```python
from build123d import *

# Parameters (mm, degrees)
F0_W          = 27
F0_H          = 27
F1_DEPTH      = 0.8
F2_D          = 2.65
F3_R          = 2
F4_W          = 5
F4_H          = 8
F4_W_2        = 8
F4_H_2        = 6
F4_R          = 0.9
F5_DEPTH      = 3
F7_DEPTH      = 2.8
F7_DEPTH_BACK = 2


with BuildPart() as f1:
    # F0 (on Top) → F1 (new body)
    with BuildSketch(Plane.XY):
        Rectangle(F0_W, F0_H)
    extrude(amount=F1_DEPTH)

    # F2 (through all)
    with Locations(Plane(origin=(0, 0, 0), x_dir=(1, 0, 0), z_dir=(0, 0, -1))):
        with Locations((-10, 10), (-10, -10), (10, 10), (10, -10)):
            Hole(F2_D / 2)

    # F3
    f3_edges = [f1.edges().sort_by_distance(p)[0] for p in [
        (-13.5, -13.5, 0.4),
        (-13.5, 13.5, 0.4),
        (13.5, -13.5, 0.4),
        (13.5, 13.5, 0.4),
    ]]
    fillet(f3_edges, radius=F3_R)

    # F4 (on face) → F5 (join)
    with BuildSketch(Plane.XY.offset(0.8)):
        with Locations((11, -1)):
            Rectangle(F4_W, F4_H)
        with Locations((1, -12.15)):
            Rectangle(F4_W_2, F4_H_2)
        with Locations((-3.5, 12)):
            Circle(F4_R)
    extrude(amount=F5_DEPTH)

    # F6 (on Top) → F7 (join, two sides)
    with BuildSketch(Plane.XY) as f7_sk:
        with BuildLine():
            Line((7, 10), (7, 13.5))
            Line((7, 13.5), (-7, 13.5))
            Line((-7, 13.5), (-7, 10))
            ThreePointArc((-7, 10), (-7.87868, 7.87868), (-10, 7))
            Line((-10, 7), (-13.5, 7))
            Line((-13.5, 7), (-13.5, -7))
            Line((-13.5, -7), (-10, -7))
            ThreePointArc((-10, -7), (-7.87868, -7.87868), (-7, -10))
            Line((-7, -10), (-7, -13.5))
            Line((-7, -13.5), (7, -13.5))
            Line((7, -13.5), (7, -10))
            ThreePointArc((7, -10), (7.87868, -7.87868), (10, -7))
            Line((10, -7), (13.5, -7))
            Line((13.5, -7), (13.5, 7))
            Line((13.5, 7), (10, 7))
            ThreePointArc((10, 7), (7.87868, 7.87868), (7, 10))
        make_face()
    extrude(amount=F7_DEPTH)
    extrude(f7_sk.sketch, amount=-F7_DEPTH_BACK)


solid = f1.part
```
Design review of the part built by this model. Coordinates are the model's own, in mm. A direction names the side the tool comes from. Coordinates: 2 decimals unless noted, no trailing zeros. Loops run counter-clockwise (first coordinate to the right, second up) from the corner with the lowest first, then second, coordinate; pieces in that order, holes last. Notation, with made-up numbers: (33.25, 87) - (76.25, 87) arc R19 cw to (76.25, 95) - close; hole circle Ø9 at (48, -16). An arc over 180 degrees is marked (long way). Use CSV: the item, a comma, the result in double quotes. Start each with the question number.
1) Consider section A-A on z = 1.15. Write out the cut boundary in (x, y).
2) Consider section C-C on y = -13. Write out the cut boundary in (x, z), then the cut area to 3 significant figures.
3) For pin 1 Ø1.6 at (x, z) = (-11, 2) entering from +Y; pin 2 Ø1.1 at (x, z) = (10.5, 3.5) entering from -Y; pin 3 Ø2.5 at (y, z) = (-12.5, 2.5) entering from -X; pin 4 Ø1.6 at (x, y) = (-10, -10) entering from +Z, all flat-tipped, find the tip position at first contact; note any pin that passes through.
4) Tool access review of faces 1 (the flat face through (-7, 12, -1)), 2 (the flat face through (11, -5, 3)), 3 (the cylindrical face through (-3.62, 12.89, 3.29)), 4 (the flat face through (12, -7, 2)): name each direction out of +Z, -Z, +X, -X, +Y, -Y from which nothing blocks a thin tool from reaching the whole face with its end or side.
5) Consider section B-B on x = -3.5. Write out the cut boundary in (y, z), then the cut area to 3 significant figures.
6) Wall thickness on L1, parallel to X at y = 10, z = 0.1 (3 decimals); L2, parallel to Y at x = 11, z = 0.75: over which ranges is each line inside the solid? List them lowest first. Write a range as from..to.
7) Consider section D-D on z = -0.7. Write out the cut boundary in (x, y), then the cut area to 3 significant figures.
Geometry says:
1,outline,"(-13.5, -7) - (-10, -7) arc R3 cw to (-7, -10) - (-7, -13.5) - (-3, -13.5) - (-3, -15.15) - (5, -15.15) - (5, -13.5) - (7, -13.5) - (7, -10) arc R3 cw to (10, -7) - (13.5, -7) - (13.5, 7) - (10, 7) arc R3 cw to (7, 10) - (7, 13.5) - (-7, 13.5) - (-7, 10) arc R3 cw to (-10, 7) - (-13.5, 7) - close"
2,outline,"(-12.82, 0) - (-7, 0) - (-7, -2) - (7, -2) - (7, 0) - (12.82, 0) - (12.82, 0.8) - (7, 0.8) - (7, 2.8) - (5, 2.8) - (5, 3.8) - (-3, 3.8) - (-3, 2.8) - (-7, 2.8) - (-7, 0.8) - (-12.82, 0.8) - close"
2,area,"84.5 mm^2"
3,pin 1,"y = 7"
3,pin 2,"y = -5"
3,pin 3,"x = -7"
3,pin 4,"through"
4,face 1,"-Z, -X, +Y"
4,face 2,"+Z, +X, -X, -Y"
4,face 3,"+Z"
4,face 4,"+Z, +X, -Y"
5,outline,"(-13.5, -2) - (13.5, -2) - (13.5, 2.8) - (12.9, 2.8) - (12.9, 3.8) - (11.1, 3.8) - (11.1, 2.8) - (-13.5, 2.8) - close"
5,area,"131 mm^2"
6,L1,"-13.5..-11.325, -8.675..8.675, 11.325..13.5"
6,L2,"-13.5..-10.87, -9.13..9.13, 10.87..13.5"
7,outline,"(-13.5, -7) - (-10, -7) arc R3 cw to (-7, -10) - (-7, -13.5) - (7, -13.5) - (7, -10) arc R3 cw to (10, -7) - (13.5, -7) - (13.5, 7) - (10, 7) arc R3 cw to (7, 10) - (7, 13.5) - (-7, 13.5) - (-7, 10) arc R3 cw to (-10, 7) - (-13.5, 7) - close"
7,area,"568 mm^2"
